Autodesk Inventor part; units mm, degrees
ref_plane "Work Plane1" through (-11.503, 4.9936, -43.1394) normal (0, 1, 0) x (1, 0, 0)
ref_plane "YZ Plane" through (0, 0, 0) normal (1, 0, 0) x (0, 1, 0)
ref_plane "XZ Plane" through (0, 0, 0) normal (0, 1, 0) x (-1, 0, 0)
sketch "Sketch1" plane through (0, 0, 0) normal (0, 1, 0) x (-1, 0, 0)
  line L0 (0, 0) -> (0, -47.0662)
  line L1 (0, -47.0662) -> (7.8486, -47.0662)
  line L2 (0, 0) -> (23.3934, 0)
  line L3 (23.3934, 0) -> (7.8486, -47.0662)
  dimension "d0" = 47.0662
  dimension "d1" = 7.8486
  dimension "d2" = 23.3934
extrude "Extrusion1" add sketch "Sketch1" along normal blind 3.236
sketch "Sketch2" plane through (0, 3.236, 0) normal (0, 1, 0) x (1, 0, 0)
  circle A0 centre (-3.6594, 3.9218) radius 2.4879
  line L0 (-23.3934, 0) -> (0, 0)
  dimension "d5" = 4.9759
  dimension "d6" = 3.9218
extrude "Extrusion2" add sketch "Sketch2" along normal blind 1.7577
ref_plane "Work Plane1" through (-11.503, 4.9936, -43.1394) normal (0, 1, 0) x (1, 0, 0)
sketch "Sketch3" plane through (-11.503, 4.9936, -43.1394) normal (0, 1, 0) x (1, 0, 0)
  point P0 (11.503, -43.1394)
pattern_linear "Rectangular Pattern2" count 6 spacing 7.8435 along (0, 0, -1) of "Extrusion2"
pattern_linear "Rectangular Pattern3" count 2 spacing 7.8435 along (-1, 0, 0) of "Extrusion2"
pattern_linear "Rectangular Pattern4" count 3 spacing 7.8435 along (0, 0, -1) of "Extrusion2", "Rectangular Pattern3"
shell "Shell1" thickness 1.4732 removed faces 1 at (-10.414, 0, -15.6887)
sketch "Sketch5" plane through (-21.3554, 1.7628, -1.4732) normal (0, -1, 0) x (1, 0, 0)
  circle A0 centre (14.3004, -14.2138) radius 2.4879
  circle A1 centre (14.3004, -22.0574) radius 2.4879
  circle A2 centre (14.3004, -29.9009) radius 2.4879
  circle A3 centre (14.3004, -14.2138) radius 3.2245
  circle A4 centre (14.3004, -22.0574) radius 3.2245
  circle A5 centre (14.3004, -29.9009) radius 3.2245
  circle A6 centre (6.4569, -6.3703) radius 2.4879
  circle A7 centre (6.4569, -6.3703) radius 3.2245
  circle A8 centre (14.3004, -6.3703) radius 2.4879
  circle A9 centre (14.3004, -6.3703) radius 3.2245
  line L0 (-2.038, 1.4732) -> (21.3554, 1.4732)
  line L1 (14.5717, -44.1198) -> (0, 0)
  line L2 (5.7322, -17.3559) -> (5.4452, -16.4868)
  line L3 (4.2905, -12.9906) -> (4.0034, -12.1215)
  arc A10 (5.7322, -17.3559) -> (4.0034, -12.1215) centre (6.4569, -14.2138) ccw
  arc A11 (5.4452, -16.4868) -> (4.2905, -12.9906) centre (6.4569, -14.2138) ccw
  line L4 (13.4975, -40.8674) -> (13.2036, -39.9775)
  line L5 (12.0893, -36.6039) -> (11.7954, -35.714)
  arc A12 (13.4975, -40.8674) -> (11.7954, -35.714) centre (14.3004, -37.7444) ccw
  arc A13 (13.2036, -39.9775) -> (12.0893, -36.6039) centre (14.3004, -37.7444) ccw
  dimension "d38" = 4.9759
  dimension "d39" = 4.9759
  dimension "d40" = 4.9759
  dimension "d42" = 6.4491
  dimension "d43" = 6.4491
  dimension "d45" = 6.4491
  dimension "d46" = 4.9759
  dimension "d47" = 6.4491
  dimension "d49" = 7.8435
  dimension "d50" = 7.8435
  dimension "d55" = 4.9759
  dimension "d56" = 6.4491
  dimension "d57" = 7.8435
  dimension "d58" = 7.8435
  dimension "d59" = 7.8435
extrude "Extrusion5" add sketch "Sketch5" along normal blind 1.7628 contours A3 | A4 | A5 | A7 | A9 | L1 A11 A10 | L1 A13 A12
sketch "Sketch7" plane through (0, 0, 0) normal (0, -1, 0) x (1, 0, 0)
  line L0 (-7.8486, -47.0662) -> (-23.3934, 0)
  line L1 (-22.6158, -2.3544) -> (-21.2169, -1.8924)
  line L2 (-17.3519, -13.5947) -> (-21.3554, -1.4732)
  line L3 (-21.2169, -1.8924) -> (-19.554, -6.9274)
  line L4 (-19.554, -6.9274) -> (-20.9529, -7.3894)
  line L5 (-22.6158, -2.3544) -> (-20.9529, -7.3894)
  line L6 (-19.9376, -10.4635) -> (-18.5387, -10.0015)
  line L7 (-18.2511, -15.5697) -> (-16.8522, -15.1077)
  line L8 (-16.8522, -15.1077) -> (-18.5387, -10.0015)
  line L9 (-19.9376, -10.4635) -> (-18.2511, -15.5697)
  line L10 (-13.7932, -29.0674) -> (-12.3943, -28.6053)
  line L11 (-12.3943, -28.6053) -> (-10.7022, -33.7286)
  line L12 (-9.5599, -37.1872) -> (-15.6232, -18.8291)
  line L13 (-12.1011, -34.1907) -> (-13.7932, -29.0674)
  line L14 (-12.1011, -34.1907) -> (-10.7022, -33.7286)
  line L15 (-11.4016, -36.3084) -> (-10.0028, -35.8464)
  line L16 (-10.0028, -35.8464) -> (-8.3101, -40.9713)
  line L17 (-8.1518, -41.4507) -> (-9.266, -38.0771)
  line L18 (-9.709, -41.4333) -> (-8.3101, -40.9713)
  line L19 (-9.709, -41.4333) -> (-11.4016, -36.3084)
  point P0 (0, 0)
extrude "Extrusion6" cut sketch "Sketch7" against normal blind 1.7577 contours L0 L6 L2 L8 L7 | L0 L15 L12 L16 L18 | L0 L10 L11 L14 | L0 L1 L2 L4
properties part number "opposite grey peice"
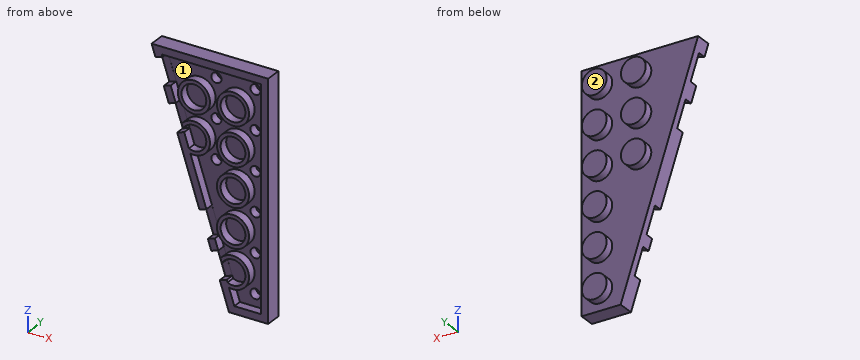
The model under review builds one solid part; all positions refer to its coordinate system, in mm. Face numbers are marked on the shaded views. A direction names the side the tool comes from. Round coordinates to 2 decimals unless told otherwise and drop trailing zeros. Put each result on its own line as item: value.
Q1. Machinability: for the marked faces 1 and 2, which of the approach directions +Z, -Z, +X, -X, +Y, -Y give a long, thin tool a straight path to every point of the face, cutting with its end or side? Answer none if there is none.
Result set:
face 1: -Y
face 2: +Z, -Z, +X, -X, +Y
Q2. For pin 1 (2 mm diameter, centred on x = -4, z = -4.5, fed in from -Y); pin 2 (1.8 mm diameter, centred on x = -3.66, z = -27.45, fed in from -Y); pin 3 (1 mm diameter, centred on y = 2, z = -15, fed in from -X); pin 4 (6 mm diameter, centred on x = -17.5, z = -36, fed in from +Y), all flat-tipped, find the tip position at first contact; note any pin that passes through.
Result set:
pin 1: stops at y = 1.76
pin 2: stops at y = 3.52
pin 3: stops at x = -18.6
pin 4: passes through
Q3. Consider section A-A, the plane y = 4.15. Count the separate pieces of the cut face and the enclosed holes in it, then the cut area to 3 significant figures.
Result set:
separate pieces: 9
enclosed holes: 0
area: 175 mm²
Q4. To check wall thickness, follow L1, parallel to X at y = 0.25, z = -31; L2, parallel to X at y = 2.65, z = -11; L3, parallel to Y at x = -3.25, z = -41. State the ranges of each line that lie inside material, in increasing order.
Result set:
L1: x = -10.26 to -9.51, -4.6 to -3.85, -1.47 to 0
L2: x = -19.76 to -12.17, -10.84 to -4.33, -2.99 to 0
L3: y = 1.76 to 4.99
